Input: dimensioned drawing with shaded views. Units: mm. Origin: part minimum x, y, z. Give positions to 0.01 mm unless a question says otherwise; leave off trailing zeros. Write each loop counter-clockwise with the first axis right and the second up, starting at its lowest first coordinate (ties: lowest second). Pieces come first, ordered by that corner, then holes.
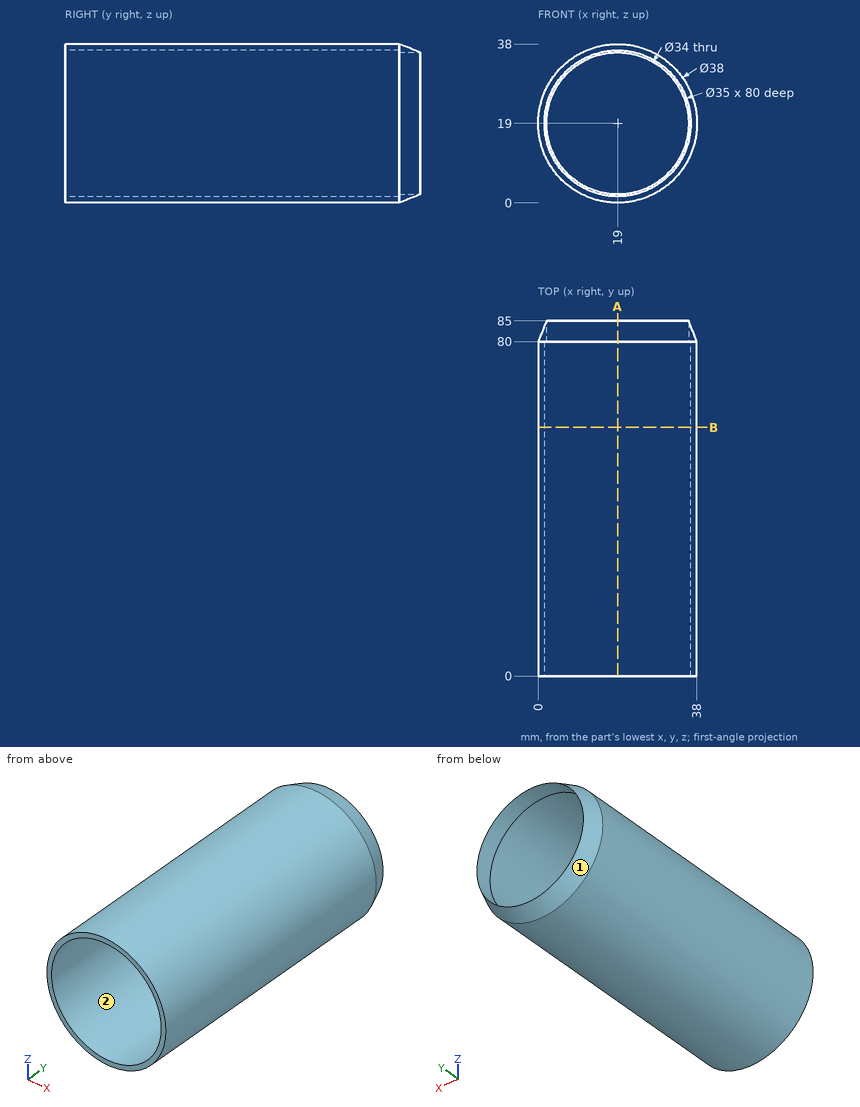
Item 1: Line query: L1, parallel to Z at x = 22, y = 76.5; L2, parallel to X at y = 9, z = 23; L3, parallel to X at y = 48, z = 35. Output: solid intervals per line, ascending.
Found:
L1: z = 0.24 to 1.76, 36.24 to 37.76
L2: x = 0.43 to 1.96, 36.04 to 37.57
L3: x = 8.75 to 11.91, 26.09 to 29.25
Item 2: Pin query (flat end, axial travel): pin 1 Ø4 at (y, z) = (42.5, 31) entering from +X; pin 2 Ø8 at (y, z) = (32, 17) entering from -X; pin 3 Ø10 at (x, y) = (27, 40.5) entering from +Z; pin 4 Ø4 at (x, y) = (18, 11.5) entering from +Z. Return the tip coordinate at first contact, or that it passes through.
Found:
pin 1: stops at x = 35.16
pin 2: stops at x = 0
pin 3: stops at z = 37.76
pin 4: stops at z = 38
Item 3: Pull-direction query (X, two-part tool) for the marked faces 1 and 2; classes: +X half, -X half, draft (parallel to the pull), parting line (faces both ways), or undercut.
Found:
face 1: parting line
face 2: undercut
Item 4: Section A-A, the plane x = 19. Return the cut outline in (y, z).
Found:
outline: (0, 0) - (80, 0) - (85, 2) - (80, 2) - (80, 1.5) - (0, 1.5) - close; (0, 36.5) - (80, 36.5) - (80, 36) - (85, 36) - (80, 38) - (0, 38) - close
Item 5: Section B-B, the plane y = 59.5. Return the cut outline in (x, z), plus the area to 3 significant figures.
Found:
outline: circle Ø38 at (19, 19); hole circle Ø35 at (19, 19)
area: 172 mm2
